from build123d import *

# Parameters (mm, degrees)
F0_R     = 25.4
F1_DEPTH = 40.2336
F2_DEPTH = 15.7734
F3_R     = 3.302


with BuildPart() as f1:
    # F0 (on Front) → F1 (new body)
    with BuildSketch(Plane.XZ):
        with BuildLine():
            ThreePointArc((-48.9148357547, -28.1233952931), (-32.0532662831, -18.3294357754), (-25.4, 0))
            ThreePointArc((-25.4, 0), (-32.0589754437, 18.3362616868), (-48.9323529412, 28.1265414802))
            ThreePointArc((-48.9323529412, 28.1265414802), (-82.5499986144, -0.0088987403), (-48.9148357547, -28.1233952931))
        make_face()
        with Locations((-53.975, 0)):
            Circle(F0_R, mode=Mode.SUBTRACT)
        with Locations((-53.975, 0)):
            Circle(F0_R)
        with BuildLine():
            ThreePointArc((-40.5617797533, -4.9211968934), (-68.262089785, 0.1082669213), (-40.488739251, 4.717353841))
            Line((-40.488739251, 4.717353841), (-36.2469597058, 4.7305268942))
            Line((-36.2469597058, 4.7305268942), (-36.3199797533, -4.9211968934))
            Line((-36.3199797533, -4.9211968934), (-40.5617797533, -4.9211968934))
        make_face(mode=Mode.SUBTRACT)
    extrude(amount=F1_DEPTH)

    # F0 (on Front) → F2 (join)
    with BuildSketch(Plane.XZ):
        with BuildLine():
            ThreePointArc((3.3617647059, -18.7510276535), (19.05, 0), (3.3617647059, 18.7510276535))
            Line((3.3617647059, 18.7510276535), (3.3617647059, 9.5877076542))
            ThreePointArc((3.3617647059, 9.5877076542), (8.2879771178, 5.8766517077), (10.16, 0))
            ThreePointArc((10.16, 0), (8.2879771178, -5.8766517077), (3.3617647059, -9.5877076542))
            Line((3.3617647059, -9.5877076542), (3.3617647059, -18.7510276535))
        make_face()
        with BuildLine():
            ThreePointArc((-48.9323529412, 28.1265414802), (-32.0589754437, 18.3362616868), (-25.4, 0))
            ThreePointArc((-25.4, 0), (-32.0532662831, -18.3294357754), (-48.9148357547, -28.1233952931))
            Line((-48.9148357547, -28.1233952931), (3.3617647059, -18.7510276535))
            Line((3.3617647059, -18.7510276535), (3.3617647059, -9.5877076542))
            ThreePointArc((3.3617647059, -9.5877076542), (-10.16, 0), (3.3617647059, 9.5877076542))
            Line((3.3617647059, 9.5877076542), (3.3617647059, 18.7510276535))
            Line((3.3617647059, 18.7510276535), (-48.9323529412, 28.1265414802))
        make_face()
    extrude(amount=F2_DEPTH)

    # F3
    f3_edges = [f1.edges().sort_by_distance(p)[0] for p in [
        (-82.55, -40.2336, 0),
    ]]
    fillet(f3_edges, radius=F3_R)


solid = f1.part
Can you work these out from the model? Positions are in its coordinate system, mm. Give positions to 0.01 mm unless a question says otherwise; leave off trailing zeros. Loops run counter-clockwise (first coordinate to the right, second up) from the corner with the lowest first, then second, coordinate; pieces in that order, holes last. Notation, with made-up numbers: (-18, 80) -> (27, 80) arc R23 cw to (27, 98) -> close; hole circle Ø5 at (-39, 60.5). An arc over 180 degrees is marked (long way). Write item = value, one per line.
1) Suppose I cut it at C-C on x = -17. Write out the boundary of the cut face in (y, z), then the cut area to 3 significant figures.
Check result:
outline = (-15.77, -22.4) -> (0, -22.4) -> (0, 22.4) -> (-15.77, 22.4) -> close
area = 707 mm2
2) Will these pins go through, and if not, where does the flat tip stop? pin 1 (1 mm diameter, centred on x = -28.5, y = -11, fed in from +Z); pin 2 (17 mm diameter, centred on x = -53.975, z = 0, fed in from -Y); pin 3 (2 mm diameter, centred on x = -37.5, y = -20.5, fed in from +Z); pin 4 (1 mm diameter, centred on x = -49.5, y = -36, fed in from +Z).
Check result:
pin_1 = 24.55
pin_2 = through
pin_3 = 24.02
pin_4 = 28.3
3) Suppose I cut it at B-B on x = 0. Write out the boundary of the cut face in (y, z).
Check result:
outline = (-15.77, -19.35) -> (0, -19.35) -> (0, -10.16) -> (-15.77, -10.16) -> close; (-15.77, 10.16) -> (0, 10.16) -> (0, 19.35) -> (-15.77, 19.35) -> close
4) I need wall thicknesses on L1, parallel to X at y = -21, z = -3; L2, parallel to X at y = -11.5, z = -3.5; L3, parallel to X at y = -12.5, z = 9. Which ranges of each line are inside material? Lowest first, please. Write a range as from..to.
Check result:
L1 = -82.39..-67.94, -36.31..-25.56
L2 = -82.33..-67.83, -36.31..-9.54, 9.54..18.73
L3 = -81.1..-65.07, -42.88..-4.71, 4.71..16.79
5) Suppose I cut it at A-A on y = -5.5. Give the number of separate pieces and of enclosed holes in the cut face, then the cut area to 3 significant figures.
Check result:
separate_pieces = 1
enclosed_holes = 2
area = 3,460 mm2
6) Thinking about a two-plate mould opening in Z: for faces 1 (the flat face through (-23.142, -7.776, -23.503)), 2 (the flat face through (-38, -20, -4.921)), 3 (the cylindrical face through (19.046, -7.776, -0.372)), 4 (the flat face through (-22.419, -7.776, 23.373)), which applies, released by +Z, released by -Z, zero draft, split by the parting line, or undercut?
Check result:
face_1 = released by -Z
face_2 = undercut
face_3 = split by the parting line
face_4 = released by +Z
